from build123d import *

# Parameters (mm, degrees)
F1_DEPTH = 31.75
F4_R     = 6.35
F5_DEPTH = 101.6
F6_R     = 16.66875
F7_DEPTH = 25.4


with BuildPart() as f1:
    # F0 (on Top) → F1 (new body)
    with BuildSketch(Plane.XY):
        Polygon((19.05, 10.998523), (0, 21.997045), (-19.05, 10.998523), (-19.05, -10.998523), (0, -21.997045), (19.05, -10.998523), align=None)
    extrude(amount=F1_DEPTH)

    # F2 (on Front) → F3 (revolve)
    with BuildSketch(Plane.XZ):
        Polygon((0, 31.75), (0, 69.85), (-9.525, 69.85), (-10.31875, 60.325), (-9.525, 60.325), (-10.31875, 50.8), (-9.525, 50.8), (-10.31875, 41.275), (-9.525, 41.275), (-10.31875, 31.75), align=None)
    revolve(axis=Axis((0, 0, 50.8), (0, 0, -1)))

    # F4 (on face) → F5 (cut)
    with BuildSketch(Plane.XY.offset(69.85)):
        Circle(F4_R)
    extrude(amount=-F5_DEPTH, mode=Mode.SUBTRACT)

    # F6 (on face) → F7 (cut)
    with BuildSketch(Plane(origin=(0, 0, 0), x_dir=(1, 0, 0), z_dir=(0, 0, -1))):
        Circle(F6_R)
    extrude(amount=-F7_DEPTH, mode=Mode.SUBTRACT)


solid = f1.part
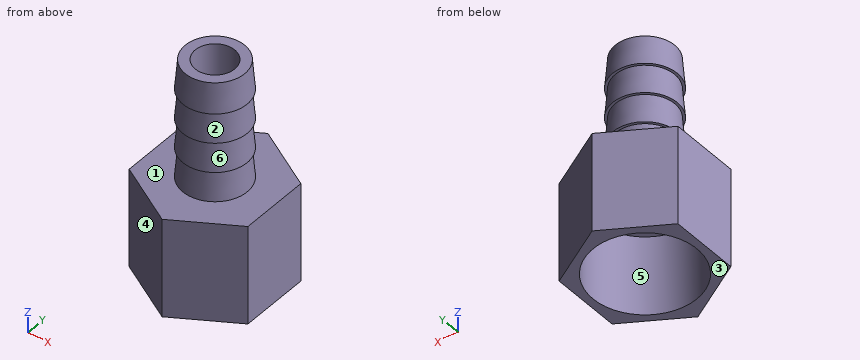
Part model, mm, in its own coordinate system. Face numbers are marked on the shaded views. A direction names the side the tool comes from. Round coordinates to 2 decimals unless told otherwise and drop trailing zeros. Write each loop counter-clockwise with the first axis right and the second up, starting at its lowest first coordinate (ties: lowest second). Pieces come first, ordered by that corner, then holes. Notation, with made-up numbers: (43, 48) - (74, 48) arc R34 ccw to (74, 80) - close; hole circle Ø11 at (-32, 74). An arc over 180 degrees is marked (long way). Use CSV: the item, a comma, the result in double quotes.
Item 1: Slice it at C-C, the plane y = 14.5. Write the cut outline in (x, z), then the cut area to 3 significant figures.
Results list:
outline,"(-12.99, 0) - (-8.22, 0) - (-8.22, 25.4) - (8.22, 25.4) - (8.22, 0) - (12.99, 0) - (12.99, 31.75) - (-12.99, 31.75) - close"
area,"407 mm²"
Item 2: Wall check: L1, parallel to Y at x = 0, z = 14.75; L2, parallel to X at y = 0, z = 19.25; L3, parallel to Z at x = 6.5, y = 5. Give the ranges that are in metal, low to high.
Results list:
L1,"y = -22 to -16.67, 16.67 to 22"
L2,"x = -19.05 to -16.67, 16.67 to 19.05"
L3,"z = 25.4 to 69.85"
Item 3: Tool access for the marked faces 4, 5 and 6: list every direction of +Z, -Z, +X, -X, +Y, -Y with a clear straight run to the whole face (end or side of a thin tool).
Results list:
face 4,"+Z, -Z, -X, -Y"
face 5,"-Z"
face 6,"none"
Item 4: Flat gauge pins, fed straight in: P1, Ø2, axis at x = 13.5, z = 18, coming from the -Y side; P2, Ø8, axis at x = 14.5, y = 15, coming from the +Z side; P3, Ø22.5, axis at x = 4.5, y = 0, coming from the -Z side. Where does each tip first touch, or does it go through?
Results list:
P1,"stops at y = -14.78"
P2,"stops at z = 31.75"
P3,"stops at z = 25.4"
Item 5: Slice it at B-B, the plane z = 63.5. Write the cut outline in (x, y).
Results list:
outline,"circle Ø20.11 at (0, 0); hole circle Ø12.7 at (0, 0)"
Item 6: Slice it at D-D, the plane x = 12.5. Write the cut outline in (y, z), then the cut area to 3 significant figures.
Results list:
outline,"(-14.78, 0) - (-11.03, 0) - (-11.03, 25.4) - (11.03, 25.4) - (11.03, 0) - (14.78, 0) - (14.78, 31.75) - (-14.78, 31.75) - close"
area,"378 mm²"
Item 7: Pull direction Z, two halves, no side cores. Call the marked faces 1, 2 and 3: pulls with the +Z half, pulls with the -Z half, needs draft (parallel to the pull), parting line crosses it, or undercut.
Results list:
face 1,"pulls with the +Z half"
face 2,"undercut"
face 3,"pulls with the -Z half"
Item 8: Slice it at A-A, the plane y = 0. Write the cut outline in (x, z) (3 decimals), then the cut area to 3 significant figures.
Results list:
outline,"(-19.05, 0) - (-16.669, 0) - (-16.669, 25.4) - (-6.35, 25.4) - (-6.35, 69.85) - (-9.525, 69.85) - (-10.319, 60.325) - (-9.525, 60.325) - (-10.319, 50.8) - (-9.525, 50.8) - (-10.319, 41.275) - (-9.525, 41.275) - (-10.319, 31.75) - (-19.05, 31.75) - close; (6.35, 25.4) - (16.669, 25.4) - (16.669, 0) - (19.05, 0) - (19.05, 31.75) - (10.319, 31.75) - (9.525, 41.275) - (10.319, 41.275) - (9.525, 50.8) - (10.319, 50.8) - (9.525, 60.325) - (10.319, 60.325) - (9.525, 69.85) - (6.35, 69.85) - close"
area,"554 mm²"
